Build history of the part. All positions in model axes, mm. A direction names the side the tool comes from. Round coordinates to 2 decimals unless told otherwise and drop trailing zeros. Order: outer loops, then holes, each group sorted by start corner. A loop starts at its lowest first (then second) coordinate and runs counter-clockwise, first axis right, second up. Notation, with made-up numbers: M -29,83.25 L 21,83.25 A26 ccw 21,115.25 Z; hole C -22,-27.5 d9. An arc over 180 degrees is marked long. Use CSV: the item, a comma, the result in double quotes.
from build123d import *

# Parameters (mm, degrees)
SKETCH1_W            = 44
SKETCH1_H            = 30
BOSS_EXTRUDE1_DEPTH  = 54.5
SKETCH5_W            = 5
SKETCH5_H            = 30
BOSS_EXTRUDE3_DEPTH  = 6.8
SKETCH9_R            = 1.3
CUT_EXTRUDE6_DEPTH   = 6
FILLET1_R            = 1.5
FILLET2_R            = 1.25
SKETCH11_W           = 34
SKETCH11_H           = 24
CUT_EXTRUDE7_DEPTH   = 51.25
SKETCH13_R           = 5
SKETCH13_R_2         = 1.3
CUT_EXTRUDE8_DEPTH   = 3.5
CIRPATTERN1_COUNT    = 8
SKETCH15_W           = 20
SKETCH15_H           = 10
CUT_EXTRUDE10_DEPTH  = 5
FILLET6_R            = 1.5
FILLET6_OF_MIRROR4_R = 1.5
SKETCH16_W           = 34
SKETCH16_H           = 11.5
SKETCH16_H_2         = 10.75
SKETCH16_H_3         = 15
CUT_EXTRUDE11_DEPTH  = 3
CHAMFER1_SIZE        = 2.75
SKETCH18_R           = 1.3
CUT_EXTRUDE12_DEPTH  = 5
FILLET7_R            = 1.5
CUT_EXTRUDE13_DEPTH  = 1


with BuildPart() as part:
    # Sketch1 → Boss-Extrude1 (new body)
    with BuildSketch(Plane(origin=(0, 0, 0), x_dir=(1, 0, 0), z_dir=(0, 1, 0))):
        with Locations((22, 15)):
            Rectangle(SKETCH1_W, SKETCH1_H)
    extrude(amount=BOSS_EXTRUDE1_DEPTH)

    # Sketch5 → Boss-Extrude3 (add)
    with BuildSketch(Plane(origin=(0, 54.5, 0), x_dir=(1, 0, 0), z_dir=(0, 1, 0))):
        with Locations((2.5, 15)):
            Rectangle(SKETCH5_W, SKETCH5_H)
    boss_extrude3 = extrude(amount=BOSS_EXTRUDE3_DEPTH)

    # Sketch9 → Cut-Extrude6 (cut, through all)
    with BuildSketch(Plane(origin=(5, 0, 0), x_dir=(0, 0, -1), z_dir=(1, 0, 0))):
        with Locations((26, 58.7)):
            Circle(SKETCH9_R)
        with Locations((4, 58.7)):
            Circle(SKETCH9_R)
    cut_extrude6 = extrude(amount=-CUT_EXTRUDE6_DEPTH, mode=Mode.SUBTRACT)

    # Mirror2: Boss-Extrude3, Cut-Extrude6 across plane
    add(boss_extrude3.mirror(Plane.ZY.offset(-22)))
    add(cut_extrude6.mirror(Plane.ZY.offset(-22)), mode=Mode.SUBTRACT)

    # Fillet1
    fillet1_edges = [part.edges().sort_by_distance(p)[0] for p in [
        (2.5, 61.3, 0),
        (2.5, 61.3, -30),
        (41.5, 61.3, -30),
        (41.5, 61.3, 0),
    ]]
    fillet(fillet1_edges, radius=FILLET1_R)

    # Fillet2
    fillet2_edges = [part.edges().sort_by_distance(p)[0] for p in [
        (22, 0, -30),
        (44, 0, -15),
        (22, 0, 0),
        (0, 0, -15),
    ]]
    fillet(fillet2_edges, radius=FILLET2_R)

    # Sketch11 → Cut-Extrude7 (cut)
    with BuildSketch(Plane(origin=(0, 54.5, 0), x_dir=(1, 0, 0), z_dir=(0, 1, 0))):
        with Locations((22, 15)):
            Rectangle(SKETCH11_W, SKETCH11_H)
    extrude(amount=-CUT_EXTRUDE7_DEPTH, mode=Mode.SUBTRACT)

    # Sketch13 → Cut-Extrude8 (cut)
    with BuildSketch(Plane.XZ):
        with Locations((22, -15)):
            Circle(SKETCH13_R)
        with Locations((33, -15)):
            Circle(SKETCH13_R_2)
    cut_extrude8 = extrude(amount=-CUT_EXTRUDE8_DEPTH, mode=Mode.SUBTRACT)

    # CirPattern1: Cut-Extrude8 ×8 about axis
    cirpattern1_axis = Axis((22, 0, -15), (0, 1, 0))
    for i in range(1, CIRPATTERN1_COUNT):
        add(cut_extrude8.rotate(cirpattern1_axis, i * 360 / CIRPATTERN1_COUNT), mode=Mode.SUBTRACT)

    # Sketch15 → Cut-Extrude10 (cut)
    with BuildSketch(Plane(origin=(44, 0, 0), x_dir=(0, 0, -1), z_dir=(1, 0, 0))):
        with Locations((15, 18.25)):
            Rectangle(SKETCH15_W, SKETCH15_H)
        with Locations((15, 40.25)):
            Rectangle(SKETCH15_W, SKETCH15_H)
    cut_extrude10 = extrude(amount=-CUT_EXTRUDE10_DEPTH, mode=Mode.SUBTRACT)

    # Fillet6
    fillet6_edges = [part.edges().sort_by_distance(p)[0] for p in [
        (41.5, 23.25, -5),
        (41.5, 13.25, -5),
        (41.5, 13.25, -25),
        (41.5, 23.25, -25),
        (41.5, 45.25, -5),
        (41.5, 35.25, -5),
        (41.5, 35.25, -25),
        (41.5, 45.25, -25),
    ]]
    fillet(fillet6_edges, radius=FILLET6_R)

    # Mirror4: Cut-Extrude10 across plane
    add(cut_extrude10.mirror(Plane.ZY.offset(-22)), mode=Mode.SUBTRACT)

    # Fillet6 of Mirror4
    fillet6_of_mirror4_edges = [part.edges().sort_by_distance(p)[0] for p in [
        (2.5, 23.25, -5),
        (2.5, 13.25, -5),
        (2.5, 13.25, -25),
        (2.5, 23.25, -25),
        (2.5, 45.25, -5),
        (2.5, 35.25, -5),
        (2.5, 35.25, -25),
        (2.5, 45.25, -25),
    ]]
    fillet(fillet6_of_mirror4_edges, radius=FILLET6_OF_MIRROR4_R)

    # Sketch16 → Cut-Extrude11 (cut)
    with BuildSketch(Plane.XY):
        with Locations((22, 9)):
            Rectangle(SKETCH16_W, SKETCH16_H)
        with Locations((22, 49.125)):
            Rectangle(SKETCH16_W, SKETCH16_H_2)
        with Locations((22, 29.25)):
            Rectangle(SKETCH16_W, SKETCH16_H_3)
    cut_extrude11 = extrude(amount=-CUT_EXTRUDE11_DEPTH, mode=Mode.SUBTRACT)

    # Mirror5: Cut-Extrude11 across plane
    add(cut_extrude11.mirror(Plane(origin=(0, 0, -15), x_dir=(1, 0, 0), z_dir=(0, 0, -1))), mode=Mode.SUBTRACT)

    # Chamfer1
    chamfer1_edges = [part.edges().sort_by_distance(p)[0] for p in [
        (39, 3.25, -15),
        (5, 3.25, -15),
    ]]
    chamfer(chamfer1_edges, length=CHAMFER1_SIZE)

    # Sketch18 → Cut-Extrude12 (cut)
    with BuildSketch(Plane.ZY):
        with Locations((-22.75, 29.25)):
            Circle(SKETCH18_R)
        with Locations((-7.25, 29.25)):
            Circle(SKETCH18_R)
        with Locations((-22.75, 9.625)):
            Circle(SKETCH18_R)
        with Locations((-7.25, 9.625)):
            Circle(SKETCH18_R)
    cut_extrude12 = extrude(amount=-CUT_EXTRUDE12_DEPTH, mode=Mode.SUBTRACT)

    # Fillet7
    fillet7_edges = [part.edges().sort_by_distance(p)[0] for p in [
        (5, 18.25, -3),
        (5, 40.25, -3),
        (39, 18.25, -3),
        (39, 40.25, -3),
        (5, 43.75, -1.5),
        (39, 43.75, -1.5),
        (5, 21.75, -1.5),
        (5, 36.75, -1.5),
        (39, 36.75, -1.5),
        (39, 21.75, -1.5),
        (39, 14.75, -1.5),
        (5, 14.75, -1.5),
        (39, 18.25, -27),
        (39, 40.25, -27),
        (5, 18.25, -27),
        (5, 40.25, -27),
        (5, 43.75, -28.5),
        (39, 43.75, -28.5),
        (5, 36.75, -28.5),
        (5, 21.75, -28.5),
        (39, 21.75, -28.5),
        (39, 36.75, -28.5),
        (5, 14.75, -28.5),
        (39, 14.75, -28.5),
    ]]
    fillet(fillet7_edges, radius=FILLET7_R)

    # Sketch19 → Cut-Extrude13 (cut)
    with BuildSketch(Plane(origin=(5, 0, 0), x_dir=(0, 0, -1), z_dir=(1, 0, 0))):
        Polygon((8.779978213, 26.6), (10.309956427, 29.25), (8.779978213, 31.9), (5.720021787, 31.9), (4.190043573, 29.25), (5.720021787, 26.6), align=None)
        Polygon((21.220021787, 26.6), (24.279978213, 26.6), (25.809956427, 29.25), (24.279978213, 31.9), (21.220021787, 31.9), (19.690043573, 29.25), align=None)
        Polygon((5.720021787, 6.975), (8.779978213, 6.975), (10.309956427, 9.625), (8.779978213, 12.275), (5.720021787, 12.275), (4.190043573, 9.625), align=None)
        Polygon((21.220021787, 6.975), (24.279978213, 6.975), (25.809956427, 9.625), (24.279978213, 12.275), (21.220021787, 12.275), (19.690043573, 9.625), align=None)
    cut_extrude13 = extrude(amount=-CUT_EXTRUDE13_DEPTH, mode=Mode.SUBTRACT)

    # Mirror6: Cut-Extrude12, Cut-Extrude13 across plane
    add(cut_extrude12.mirror(Plane.ZY.offset(-22)), mode=Mode.SUBTRACT)
    add(cut_extrude13.mirror(Plane.ZY.offset(-22)), mode=Mode.SUBTRACT)


solid = part.part
(1) Cut at A-A, the plane y = 42. Give the cut face in (x, z), and give its area (3 significant figures).
Answer block:
outline,"M 0,-30 L 44,-30 L 44,-25 L 39,-25 L 39,-25.5 A1.5 cw 37.5,-27 L 6.5,-27 A1.5 cw 5,-25.5 L 5,-25 L 0,-25 Z; M 0,-5 L 5,-5 L 5,-4.5 A1.5 cw 6.5,-3 L 37.5,-3 A1.5 cw 39,-4.5 L 39,-5 L 44,-5 L 44,0 L 0,0 Z"
area,"306 mm²"
(2) Drop flat-ended pins along their axis: pin 1 (3.5 mm diameter, centred on x = 24.5, y = 18, fed in from +Z); pin 2 (3 mm diameter, centred on x = 8.5, z = -3.5, fed in from +Y). Give the stop position or say it passes through.
Answer block:
pin 1,"stops at z = 0"
pin 2,"stops at y = 43.75"
(3) Tool access for faces 1 (the face through (38.55, 14.32, -1.78)), 2 (the face through (5.43, 44.2, -1.78)), 3 (the face through (39.493, 10.931, -25.056)): list every direction of +Z, -Z, +X, -X, +Y, -Y with a clear straight run to the whole face (end or side of a thin tool).
Answer block:
face 1,"+Z, -Z"
face 2,"+Z, -Z, +Y"
face 3,"none"
(4) Cut at D-D, the plane x = 33. Give the cut face in (y, z), and give its area (3 significant figures).
Answer block:
outline,"M 0,-28.75 A1.25 ccw 1.25,-30 L 3.25,-30 L 3.25,-16.3 L 0,-16.3 Z; M 0,-13.7 L 3.25,-13.7 L 3.25,0 L 1.25,0 A1.25 ccw 0,-1.25 Z; M 14.75,-30 L 21.75,-30 L 21.75,-27 L 14.75,-27 Z; M 14.75,-3 L 21.75,-3 L 21.75,0 L 14.75,0 Z; M 36.75,-30 L 43.75,-30 L 43.75,-27 L 36.75,-27 Z; M 36.75,-3 L 43.75,-3 L 43.75,0 L 36.75,0 Z"
area,"172 mm²"
(5) Cut at C-C, the plane y = 58.7. Give the cut face in (x, z).
Answer block:
outline,"M 0,-30 L 5,-30 L 5,-27.3 L 0,-27.3 Z; M 0,-24.7 L 5,-24.7 L 5,-5.3 L 0,-5.3 Z; M 0,-2.7 L 5,-2.7 L 5,0 L 0,0 Z; M 39,-30 L 44,-30 L 44,-27.3 L 39,-27.3 Z; M 39,-24.7 L 44,-24.7 L 44,-5.3 L 39,-5.3 Z; M 39,-2.7 L 44,-2.7 L 44,0 L 39,0 Z"
(6) Two-plate mould, pull along X, no slides. Class faces 4 (the face through (41.46, 44.8, -5.43)), 5 (the face through (5.43, 40.18, -26.55)): released by +X, released by -X, zero draft, split by the parting line, or undercut.
Answer block:
face 4,"zero draft"
face 5,"undercut"
(7) Wall check: line 1 (Y direction, x = 1.25, z = -7.25) (3 decimals); line 2 (Y direction, x = 39.5, z = -15.5); line 3 (X direction, y = 57, z = -24.75). Give the ranges that are in metal, low to high. Write a range as from..to.
Answer block:
line 1,"y = 0..8.325, 10.925..13.25, 23.25..27.95, 30.55..35.25, 45.25..61.3"
line 2,"y = 0..13.25, 23.25..35.25, 45.25..61.3"
line 3,"x = 0..5, 39..44"
(8) Cut at B-B, the plane x = 22. Count the separate pieces of the cut face and the enclosed holes in it, and give its area (3 significant figures).
Answer block:
separate pieces,"8"
enclosed holes,"0"
area,"131 mm²"
